Could you check a few things on this model? Use its own coordinates, in mm. A direction names the side the tool comes from. Give positions to 0.01 mm unless a question says otherwise; leave off trailing zeros. Loops run counter-clockwise (first coordinate to the right, second up) from the corner with the lowest first, then second, coordinate; pieces in that order, holes last. Notation, with made-up numbers: M 54,-21 L 60,-21 A13 ccw 60,-8 Z; hole C 54.25,80.5 d5. An arc over 180 degrees is marked long. Answer in a Markdown table with one row per item. Add a question column.
```python
from build123d import *

# Parameters (mm, degrees)
SKETCH1_R           = 22
SKETCH1_R_2         = 16
BOSS_EXTRUDE2_DEPTH = 7
SKETCH3_R           = 24
BOSS_EXTRUDE6_DEPTH = 9
SKETCH6_R           = 32
BOSS_EXTRUDE7_DEPTH = 9
SKETCH7_R           = 16
CUT_EXTRUDE2_DEPTH  = 56.425625842
CUT_EXTRUDE3_DEPTH  = 79.383671769
SKETCH9_R           = 3
CUT_EXTRUDE4_DEPTH  = 56.036351623


with BuildPart() as part:
    # Sketch1 → Boss-Extrude2 (new, symmetric)
    with BuildSketch(Plane.XY):
        Circle(SKETCH1_R)
        Circle(SKETCH1_R_2, mode=Mode.SUBTRACT)
    extrude(amount=BOSS_EXTRUDE2_DEPTH, both=True)

    # Sketch3 → Boss-Extrude6 (add)
    with BuildSketch(Plane.XY.offset(7)):
        Circle(SKETCH3_R)
    extrude(amount=BOSS_EXTRUDE6_DEPTH)

    # Sketch6 → Boss-Extrude7 (add)
    with BuildSketch(Plane.XY.offset(16)):
        Circle(SKETCH6_R)
    extrude(amount=BOSS_EXTRUDE7_DEPTH)

    # Sketch7 → Cut-Extrude2 (cut, through all)
    with BuildSketch(Plane(origin=(0, 0, -7), x_dir=(-1, 0, 0), z_dir=(0, 0, -1))):
        Circle(SKETCH7_R)
    extrude(amount=-CUT_EXTRUDE2_DEPTH, mode=Mode.SUBTRACT)

    # Mirror3: part across plane


with BuildPart() as part_1:
    add(part.part)
    add(part.part.mirror(Plane.XY.offset(-7)))

    # Sketch8 → Cut-Extrude3 (cut, through all)
    with BuildSketch(Plane.XY.offset(25)):
        Polygon((-194.543052514, 0), (-35.372068519, 0), (34.570182834, 0), (193.741166829, 0), (193.741166829, -318.34196799), (-194.543052514, -318.34196799), align=None)
    extrude(amount=-CUT_EXTRUDE3_DEPTH, mode=Mode.SUBTRACT)

    # Sketch9 → Cut-Extrude4 (cut, through all)
    with BuildSketch(Plane(origin=(0, 22, 0), x_dir=(1, 0, 0), z_dir=(0, 1, 0))):
        with Locations(Location((0, 7, 0), (0, 0, 270))):
            Circle(SKETCH9_R)
    extrude(amount=-CUT_EXTRUDE4_DEPTH, mode=Mode.SUBTRACT)


solid = part_1.part
```
Item 1: For faces 4 (the face through (0, 27, 16)), 5 (the face through (0.704, 31.992, 20.437)), which set-ups out of +Z, -Z, +X, -X, +Y, -Y let a thin tool reach every point of the face, with its end or its side?
Item 2: Suppose I cut it at A-A (x = 0). List the corners of the cut face in (y, z) for me, then the cut area to 3 significant figures.
Item 3: If we mould it in two halves opening along Z, with no side actions, what happens to faces 1 (the face through (-0.4, 16.2, -39)), 2 (the face through (0.528, 23.994, 11.437)), 3 (the face through (0.704, 31.992, -34.437))? For each: +Z half, -Z half, draft (parallel to the pull), parting line (faces both ways), or undercut.
Item 4: Suppose I cut it at B-B (y = 29.5). List the corners of the cut face in (x, z) for me, then the cut area to 3 significant figures.
Item 5: For P1, Ø1, axis at x = 13, z = -1.5, coming from the +Y side; P2, Ø3, axis at y = 6.5, z = -24, coming from the +X side; P3, Ø4, axis at x = -4, z = -10, coming from the -Y side, each with a flat end and sliding along its axis, tell me the tip position at first contact or that it passes through.
Item 6: Suppose I cut it at C-C (y = 19). List the corners of the cut face in (x, z) for me, then the cut area to 3 significant figures.
Item 7: Suppose I cut it at D-D (z = -33.5). List the corners of the cut face in (x, y) for me, then the cut area to 3 significant figures.
Item 8: I need wall thicknesses on L1, parallel to Z at x = 0, y = 17.5; L2, parallel to Z at x = 1.5, y = 22; L3, parallel to X at y = 8, z = 18.5. Which ranges of each line are inside material? Lowest first, please.
Values found:
| question | item | result |
|---|---|---|
| 1 | face 4 | +Y |
| 1 | face 5 | +Z, -Z, +Y |
| 2 | outline | M 16,-39 L 32,-39 L 32,-30 L 24,-30 L 24,-21 L 22,-21 L 22,-10 L 16,-10 Z; M 16,-4 L 22,-4 L 22,7 L 24,7 L 24,16 L 32,16 L 32,25 L 16,25 Z |
| 2 | area | 564 mm² |
| 3 | face 1 | -Z half |
| 3 | face 2 | undercut |
| 3 | face 3 | draft |
| 4 | outline | M -12.4,-39 L 12.4,-39 L 12.4,-30 L -12.4,-30 Z; M -12.4,16 L 12.4,16 L 12.4,25 L -12.4,25 Z |
| 4 | area | 446 mm² |
| 5 | P1 | y = 18.1 |
| 5 | P2 | x = 23.47 |
| 5 | P3 | y = 14.83 |
| 6 | outline | M -25.75,-39 L 25.75,-39 L 25.75,-30 L 14.66,-30 L 14.66,-21 L 11.09,-21 L 11.09,7 L 14.66,7 L 14.66,16 L 25.75,16 L 25.75,25 L -25.75,25 L -25.75,16 L -14.66,16 L -14.66,7 L -11.09,7 L -11.09,-21 L -14.66,-21 L -14.66,-30 L -25.75,-30 Z; hole C 0,-7 d6 |
| 6 | area | 2,050 mm² |
| 7 | outline | M -32,0 L -16,0 A16 cw 16,0 L 32,0 A32 ccw Z |
| 7 | area | 1,210 mm² |
| 8 | L1 | -39 to -10, -4 to 25 |
| 8 | L2 | -39 to -21, 7 to 25 |
| 8 | L3 | -30.98 to -13.86, 13.86 to 30.98 |
